Part model, mm, in its own coordinate system. A direction names the side the tool comes from. Round coordinates to 2 decimals unless told otherwise and drop trailing zeros. Write each loop counter-clockwise with the first axis right and the second up, starting at its lowest first coordinate (ties: lowest second). Pieces come first, ordered by that corner, then holes.
```python
from build123d import *

# Parameters (mm, degrees)
SKETCH1_R           = 1.5
SKETCH1_R_2         = 4
BOSS_EXTRUDE2_DEPTH = 3


with BuildPart() as part:
    # Sketch1 → Boss-Extrude2 (new body)
    with BuildSketch(Plane(origin=(0, 0, 0), x_dir=(1, 0, 0), z_dir=(0, 1, 0))):
        with BuildLine():
            Line((-43, 65.026712015), (-25.898177638, 65.026712015))
            Line((-25.898177638, 65.026712015), (-25.898177638, 27.526712015))
            ThreePointArc((-25.898177638, 27.526712015), (-25.165944591, 25.758945062), (-23.398177638, 25.026712015))
            Line((-23.398177638, 25.026712015), (31.601822362, 25.026712015))
            ThreePointArc((31.601822362, 25.026712015), (33.369636089, 25.758964437), (34.101888511, 27.526778164))
            Line((34.101888511, 27.526778164), (34.101888511, 65.008591724))
            Line((34.101888511, 65.008591724), (42.973532608, 65.008591724))
            Line((42.973532608, 65.008591724), (42.973532608, 50.008591724))
            Line((42.973532608, 50.008591724), (39.974710246, 50.008591724))
            Line((39.974710246, 50.008591724), (39.974710246, 16.608591724))
            Line((39.974710246, 16.608591724), (42.974710246, 16.608591724))
            Line((42.974710246, 16.608591724), (42.974710246, -6.591408276))
            Line((42.974710246, -6.591408276), (39.974710246, -6.591408276))
            Line((39.974710246, -6.591408276), (39.974710246, -49.991408276))
            Line((39.974710246, -49.991408276), (42.974710246, -49.991408276))
            Line((42.974710246, -49.991408276), (42.974710246, -59.991408276))
            Line((42.974710246, -59.991408276), (15.954710246, -59.991408276))
            Line((15.954710246, -59.991408276), (15.954710246, -50.391457529))
            Line((15.954710246, -50.391457529), (17.204695418, -50.391457529))
            Line((17.204695418, -50.391457529), (17.204695418, -48.200049254))
            Line((17.204695418, -48.200049254), (15.979985173, -48.200049254))
            Line((15.979985173, -48.200049254), (15.979985173, -43.200049254))
            Line((15.979985173, -43.200049254), (12.779985173, -43.200049254))
            Line((12.779985173, -43.200049254), (12.779985173, -48.200049254))
            Line((12.779985173, -48.200049254), (11.529985173, -48.200049254))
            Line((11.529985173, -48.200049254), (11.529985173, -50.400049254))
            Line((11.529985173, -50.400049254), (12.779985173, -50.400049254))
            Line((12.779985173, -50.400049254), (12.779985173, -60.000049254))
            Line((12.779985173, -60.000049254), (-12.780014827, -60.000049254))
            Line((-12.780014827, -60.000049254), (-12.780014827, -50.400049254))
            Line((-12.780014827, -50.400049254), (-11.530014827, -50.400049254))
            Line((-11.530014827, -50.400049254), (-11.530014827, -48.200049254))
            Line((-11.530014827, -48.200049254), (-12.780014827, -48.200049254))
            Line((-12.780014827, -48.200049254), (-12.780014827, -43.200049254))
            Line((-12.780014827, -43.200049254), (-15.980014827, -43.200049254))
            Line((-15.980014827, -43.200049254), (-15.980014827, -48.200049254))
            Line((-15.980014827, -48.200049254), (-17.230014827, -48.200049254))
            Line((-17.230014827, -48.200049254), (-17.230014827, -50.400049254))
            Line((-17.230014827, -50.400049254), (-15.980014827, -50.400049254))
            Line((-15.980014827, -50.400049254), (-15.980014827, -60.000049254))
            Line((-15.980014827, -60.000049254), (-43, -60.028356008))
            Line((-43, -60.028356008), (-43, -50))
            Line((-43, -50), (-40, -50))
            Line((-40, -50), (-40, -6.6))
            Line((-40, -6.6), (-43, -6.6))
            Line((-43, -6.6), (-43, 16.6))
            Line((-43, 16.6), (-40, 16.626712015))
            Line((-40, 16.626712015), (-40, 50.026712015))
            Line((-40, 50.026712015), (-43, 50.026712015))
            Line((-43, 50.026712015), (-43, 65.026712015))
        make_face()
        with Locations(Location((-41, 5, 0), (0, 0, 270))):
            Circle(SKETCH1_R, mode=Mode.SUBTRACT)
        with Locations(Location((-36.703, 59.285, 0), (0, 0, 270))):
            Circle(SKETCH1_R, mode=Mode.SUBTRACT)
        with Locations(Location((36.703, 59.285, 0), (0, 0, 270))):
            Circle(SKETCH1_R, mode=Mode.SUBTRACT)
        with Locations(Location((-36.703, -0.405, 0), (0, 0, 270))):
            Circle(SKETCH1_R, mode=Mode.SUBTRACT)
        with Locations(Location((36.703, -0.405, 0), (0, 0, 270))):
            Circle(SKETCH1_R, mode=Mode.SUBTRACT)
        with Locations(Location((-25, -50.405, 0), (0, 0, 270))):
            Circle(SKETCH1_R_2, mode=Mode.SUBTRACT)
        with Locations(Location((25, -50.400049254, 0), (0, 0, 270))):
            Circle(SKETCH1_R_2, mode=Mode.SUBTRACT)
        with Locations(Location((41.13223265, 5, 0), (0, 0, 270))):
            Circle(SKETCH1_R, mode=Mode.SUBTRACT)
        with BuildLine():
            Line((0, -40.405), (27.5, -40.405))
            ThreePointArc((27.5, -40.405), (29.267766953, -39.672766953), (30, -37.905))
            Line((30, -37.905), (30, 17.095))
            ThreePointArc((30, 17.095), (29.267766953, 18.862766953), (27.5, 19.595))
            Line((27.5, 19.595), (0, 19.595))
            Line((0, 19.595), (-27.5, 19.595))
            ThreePointArc((-27.5, 19.595), (-29.267766953, 18.862766953), (-30, 17.095))
            Line((-30, 17.095), (-30, -37.905))
            ThreePointArc((-30, -37.905), (-29.267766953, -39.672766953), (-27.5, -40.405))
            Line((-27.5, -40.405), (0, -40.405))
        make_face(mode=Mode.SUBTRACT)
    extrude(amount=BOSS_EXTRUDE2_DEPTH)


solid = part.part
```
Q1. Cut at A-A on z = -5. Write the cut outline in (x, y).
Values follow:
outline: (-43, 0) - (-42.5, 0) - (-42.5, 3) - (-43, 3) - close; (-39.5, 0) - (-30, 0) - (-30, 3) - (-39.5, 3) - close; (30, 0) - (39.63, 0) - (39.63, 3) - (30, 3) - close; (42.63, 0) - (42.97, 0) - (42.97, 3) - (42.63, 3) - close
Q2. Cut at C-C on z = -53. Write the cut outline in (x, y).
Values follow:
outline: (-43, 0) - (-25.9, 0) - (-25.9, 3) - (-43, 3) - close; (34.1, 0) - (42.97, 0) - (42.97, 3) - (34.1, 3) - close
Q3. Drop flat-ended pins along their axis: pin 1 (1.5 mm diameter, centred on y = 1.5, z = 30.5, fed in from +X); pin 2 (0.9 mm diameter, centred on x = 41, y = 1, fed in from -Z); pin 3 (0.9 mm diameter, centred on x = -2, y = 2, fed in from +Z). Give the stop position or say it passes through.
Values follow:
pin 1: stops at x = 39.97
pin 2: stops at z = -65.01
pin 3: stops at z = 60
Q4. Mould opens along X. For faces 1 (the flat face through (0, 1, 40.405)), 2 (the flat face through (42.975, 1, 55)), 3 (the flat face through (-32, 3, 6)) say: +X half, -X half, draft (parallel to the pull), parting line (faces both ways), or undercut.
Values follow:
face 1: undercut
face 2: +X half
face 3: draft
Q5. Cut at B-B on z = 35.5. Write the cut outline in (x, y).
Values follow:
outline: (-40, 0) - (-30, 0) - (-30, 3) - (-40, 3) - close; (30, 0) - (39.97, 0) - (39.97, 3) - (30, 3) - close
Q6. Cut at D-D on y = 0.5. State how many separate pieces and enclosed holes the cut face has, plus the area to 3 significant figures.
Values follow:
separate pieces: 1
enclosed holes: 9
area: 4,040 mm2
Q7. Wall check: L1, parallel to X at y = 1, z = -5; L2, parallel to Z at x = 17, y = 2.8 (3 decimals); L3, parallel to Z at x = -3.5, y = 2.9 (3 decimals). Give the ranges that are in metal, low to high.
Values follow:
L1: x = -43 to -42.5, -39.5 to -30, 30 to 39.63, 42.63 to 42.97
L2: z = -25.027 to -19.595, 40.405 to 48.2, 50.391 to 59.991
L3: z = -25.027 to -19.595, 40.405 to 60
Q8. Which spindle directions (+Z, -Z, +X, -X, +Y, -Y) get a long thin tool onto all of the face, cutting with end or side? Do faces 4 (the cylindrical face through (-29.25, 1.48, -18.88)), 5 (the flat face through (-12.78, 1, 55)), 6 (the flat face through (4, 1, -25.027)), 7 (the flat face through (41, 1, 49.991)). Say none if no direction does.
Values follow:
face 4: +Y, -Y
face 5: +Z, +Y, -Y
face 6: -Z, +Y, -Y
face 7: +X, +Y, -Y
